Check sheet for the modelled part. Datum: model origin and axes. Units: mm. A direction names the side the tool comes from. Round coordinates to 2 decimals unless told otherwise and drop trailing zeros. Order: outer loops, then holes, each group sorted by start corner. A loop starts at its lowest first (then second) coordinate and runs counter-clockwise, first axis right, second up.
(1) Thickness scan on probe 1 along X at (y, z) = (-12, 0); probe 2 along Z at (x, y) = (-15, 12.75); probe 3 along Y at (x, z) = (12, 0.5). Record the ranges inside material, lowest first.
(2) Sectioned sample at A-A, the plane x = 10. Enter the section's corners in (y, z).
(3) Mould release check, pull along Z, two halves, no side actions. Record for faces 1 (the flat face through (0, -12, 5)), 2 (the flat face through (-20, -10, 0)), 3 (the cylindrical face through (-13.925, -9.883, -1.686)): released by +Z, released by -Z, zero draft, split by the parting line, or undercut.
(4) Depth check by flat-ended pin: pin 1 (10 mm diameter, centred on x = 9, y = -1, fed in from -Z); pin 2 (5.5 mm diameter, centred on x = 18.5, y = -2, fed in from +Z); pin 3 (4 mm diameter, centred on y = -1.5, z = -3, fed in from -X); pin 4 (3 mm diameter, centred on x = -15, z = 0, fed in from +Y). Enter the tip coordinate at first touch or a pass-through.
(5) Sectioned sample at D-D, the plane z = -1.5. Count the separate pieces of the cut face and the enclosed holes in it, and give its area (3 significant figures).
(6) Sectioned sample at B-B, the plane x = -15. Enter the section's corners in (y, z).
(7) Tool access check on faces 4 (the flat face through (-13.15, 5.333, -1.181)), 5 (the flat face through (17, 0, 0)), 6 (the flat face through (13, 5, 1)), 7 (the cylindrical face through (0.75, 10.1, 0.34)), 8 (the flat face through (-13.15, -4.863, -1.181)). Record the directions out of +Z, -Z, +X, -X, +Y, -Y that give a thin tool (end or side, any length) a straight path to the whole face; none if there is none.
(8) Sectioned sample at C-C, the plane y = 12.25. Enter the section's corners in (x, z).
```python
from build123d import *

# Parameters (mm, degrees)
BOX002_W               = 10
BOX002_H               = 10
BOX002_DEPTH           = 5
CYLINDER003_R          = 2
CYLINDER003_DEPTH      = 30
CYLINDER003_ROLL_ANGLE = -90
CYLINDER004_R          = 10
CYLINDER004_DEPTH      = 20
BOX003_W               = 15
BOX003_H               = 10
BOX003_DEPTH           = 20
FUSION001_ROLL_ANGLE   = 11.25
BOX001_W               = 10
BOX001_H               = 10
BOX001_DEPTH           = 10
BOX_W                  = 40
BOX_H                  = 30
BOX_DEPTH              = 10


with BuildPart() as cube002:
    # Box002 → Box002 (new body)
    with BuildSketch(Plane(origin=(10, -5, 0), x_dir=(1, 0, 0), z_dir=(0, 0, 1))):
        with Locations((5, 5)):
            Rectangle(BOX002_W, BOX002_H)
    extrude(amount=BOX002_DEPTH)


with BuildPart() as cylinder003:
    # Cylinder003 → Cylinder003 (new body)
    with BuildSketch(Plane.XY):
        Circle(CYLINDER003_R)
    extrude(amount=CYLINDER003_DEPTH)


with BuildPart() as cylinder003_1:
    # Cylinder003 roll: moved
    add(cylinder003.part.rotate(Axis((0, 0, 0), (1, 0, 0)), CYLINDER003_ROLL_ANGLE))


with BuildPart() as cylinder003_2:
    # Cylinder003 placement: moved
    add(cylinder003_1.part.moved(Location((-15, -15, 0))))


with BuildPart() as rail_cylinder:
    # Cylinder004 → Cylinder004 (new body)
    with BuildSketch(Plane.XY.offset(-10)):
        Circle(CYLINDER004_R)
    extrude(amount=CYLINDER004_DEPTH)


with BuildPart() as fusion001:
    # Box003 → Box003 (new body)
    with BuildSketch(Plane(origin=(-20, -5, -10), x_dir=(1, 0, 0), z_dir=(0, 0, 1))):
        with Locations((7.5, 5)):
            Rectangle(BOX003_W, BOX003_H)
    extrude(amount=BOX003_DEPTH)

    # Fusion001: union Rail Cylinder
    add(rail_cylinder.part)


with BuildPart() as fusion001_1:
    # Fusion001 roll: moved
    add(fusion001.part.rotate(Axis((0, 0, 0), (1, 0, 0)), FUSION001_ROLL_ANGLE))


with BuildPart() as fusion001_2:
    # Fusion001 placement: moved
    add(fusion001_1.part)


with BuildPart() as negative_fusion:
    # Box001 → Box001 (new body)
    with BuildSketch(Plane(origin=(5, -5, -5), x_dir=(1, 0, 0), z_dir=(0, 0, 1))):
        with Locations((5, 5)):
            Rectangle(BOX001_W, BOX001_H)
    extrude(amount=BOX001_DEPTH)

    # Fusion: union Cube002, Cylinder003, Fusion001
    add(cube002.part)
    add(cylinder003_2.part)
    add(fusion001_2.part)


with BuildPart() as cut:
    # Box → Box (new body)
    with BuildSketch(Plane(origin=(-20, -15, -5), x_dir=(1, 0, 0), z_dir=(0, 0, 1))):
        with Locations((20, 15)):
            Rectangle(BOX_W, BOX_H)
    extrude(amount=BOX_DEPTH)

    # Cut: cut Negative Fusion
    add(negative_fusion.part, mode=Mode.SUBTRACT)


solid = cut.part
```
Derived:
1. probe 1: x = -20 to -17, -13 to 20
1. probe 2: z = -5 to -2, 2 to 5
1. probe 3: y = -15 to -5, 5 to 15
2. outline: (-15, -5) - (-5, -5) - (-5, 5) - (-15, 5) - close; (5, -5) - (15, -5) - (15, 5) - (5, 5) - close
3. face 1: released by +Z
3. face 2: zero draft
3. face 3: undercut
4. pin 1: stops at z = -5
4. pin 2: stops at z = 0
4. pin 3: stops at x = 15
4. pin 4: passes through
5. separate pieces: 3
5. enclosed holes: 0
5. area: 667 mm2
6. outline: (-15, -5) - (-4.1, -5) - (-4.7, -2) - (-15, -2) - close; (-15, 2) - (-5.5, 2) - (-6.09, 5) - (-15, 5) - close; (4.1, 5) - (4.7, 2) - (15, 2) - (15, 5) - close; (5.5, -2) - (6.09, -5) - (15, -5) - (15, -2) - close
7. face 4: -Z, -X
7. face 5: +Z, +X, -X
7. face 6: +Z
7. face 7: -Z
7. face 8: +Z, -X
8. outline: (-20, -5) - (20, -5) - (20, 5) - (-20, 5) - close; hole circle Ø4 at (-15, 0)
